```python
from build123d import *

# Parameters (mm, degrees)
F1_DEPTH = 5
F2_W     = 10
F2_H     = 4
F3_DEPTH = 25
F4_R     = 5
F5_R     = 5


with BuildPart() as f1:
    # F0 (on Front) → F1 (new body)
    with BuildSketch(Plane.XZ):
        with BuildLine():
            Line((-60, -80), (-60, 0))
            Line((-60, 0), (0, 0))
            Line((0, 0), (60, 0))
            Line((60, 0), (60, -80))
            ThreePointArc((60, -80), (62.5, -82.5), (65, -80))
            Line((65, -80), (65, 8))
            Line((65, 8), (60, 8))
            Line((60, 8), (43, 8))
            Line((43, 8), (43, 32.420063))
            ThreePointArc((43, 32.420063), (40.5, 34.920063), (38, 32.420063))
            Line((38, 32.420063), (38, 15.420063))
            Line((38, 15.420063), (35.5, 15.420063))
            Line((35.5, 15.420063), (35.5, 8))
            Line((35.5, 8), (0, 8))
            Line((0, 8), (-35.5, 8))
            Line((-35.5, 8), (-35.5, 15.420063))
            Line((-35.5, 15.420063), (-38, 15.420063))
            Line((-38, 15.420063), (-38, 32.420063))
            ThreePointArc((-38, 32.420063), (-40.5, 34.920063), (-43, 32.420063))
            Line((-43, 32.420063), (-43, 8))
            Line((-43, 8), (-60, 8))
            Line((-60, 8), (-65, 8))
            Line((-65, 8), (-65, -80))
            ThreePointArc((-65, -80), (-62.5, -82.5), (-60, -80))
        make_face()
    extrude(amount=F1_DEPTH)

    # F2 (on Front) → F3 (cut)
    with BuildSketch(Plane.XZ):
        with Locations((0, 8)):
            Rectangle(F2_W, F2_H)
    extrude(amount=F3_DEPTH, mode=Mode.SUBTRACT)

    # F4
    f4_edges = [f1.edges().sort_by_distance(p)[0] for p in [
        (-65, -2.5, 8),
        (65, -2.5, 8),
    ]]
    fillet(f4_edges, radius=F4_R)

    # F5
    f5_edges = [f1.edges().sort_by_distance(p)[0] for p in [
        (-43, -2.5, 8),
        (43, -2.5, 8),
    ]]
    fillet(f5_edges, radius=F5_R)


solid = f1.part
```
Geometry: final body of the model. Coordinates: model frame, mm. A direction names the side the tool comes from. Give positions to 0.01 mm unless a question says otherwise; leave off trailing zeros. Write each loop counter-clockwise with the first axis right and the second up, starting at its lowest first coordinate (ties: lowest second). Pieces come first, ordered by that corner, then holes.
1. Reachability of faces 4 (the flat face through (-54, -2, 8)), 5 (the flat face through (54, -2, 8)), 6 (the flat face through (-60, -2, -41)), 7 (the flat face through (-65, -2, -38)), 8 (the flat face through (35.5, -2, 12)) from +Z, -Z, +X, -X, +Y, -Y: full face, straight path, thin tool, end or side. Return the list, or none.
2. Section query B-B, the plane y = -3.2. Return loops of the section in (x, z).
3. Section query A-A, the plane z = -34. Return loops of the section in (x, y), then the cut area to 3 significant figures.
4. Section query D-D, the plane x = 62.5. Return loops of the section in (y, z), then the cut area to 3 significant figures.
5. Line query: probe 1 along X at (y, z) = (-4.2, -60); probe 2 along X at (y, z) = (-3.8, 19); probe 3 along Z at (x, y) = (-19, -2.25). Output: solid intervals per line, ascending.
6. Section query C-C, the plane x = -52. Return loops of the section in (y, z), then the cut area to 3 significant figures.
7. Draft query along Y for faces 1 (the flat face through (0, 0, 3)), 2 (the flat face through (0, -2, 6)), 3 (the flat face through (0, -5, 3)). Return one class per face: released by +Y, released by -Y, zero draft, split by the parting line, or undercut.
8. Pin query (flat end, axial travel): P1, Ø2.5, axis at x = 1.5, y = -2.5, coming from the +Z side; P2, Ø2, axis at y = -2, z = 13, coming from the -X side; P3, Ø2.5, axis at y = -3.5, z = 18, coming from the -X side. Return the tip coordinate at first contact, or that it passes through.
Computed:
1. face 4: +Z, -X, +Y, -Y
1. face 5: +Z, +X, +Y, -Y
1. face 6: -Z, +Y, -Y
1. face 7: +Z, -Z, -X, +Y, -Y
1. face 8: +Z, +Y, -Y
2. outline: (-65, -80) arc R2.5 ccw to (-60, -80) - (-60, 0) - (60, 0) - (60, -80) arc R2.5 ccw to (65, -80) - (65, 3) arc R5 ccw to (60, 8) - (48, 8) arc R5 cw to (43, 13) - (43, 32.42) arc R2.5 ccw to (38, 32.42) - (38, 15.42) - (35.5, 15.42) - (35.5, 8) - (5, 8) - (5, 6) - (-5, 6) - (-5, 8) - (-35.5, 8) - (-35.5, 15.42) - (-38, 15.42) - (-38, 32.42) arc R2.5 ccw to (-43, 32.42) - (-43, 13) arc R5 cw to (-48, 8) - (-60, 8) arc R5 ccw to (-65, 3) - close
3. outline: (-65, -5) - (-60, -5) - (-60, 0) - (-65, 0) - close; (60, -5) - (65, -5) - (65, 0) - (60, 0) - close
3. area: 50.0 mm2
4. outline: (-5, -82.5) - (0, -82.5) - (0, 7.33) - (-5, 7.33) - close
4. area: 449 mm2
5. probe 1: x = -65 to -60, 60 to 65
5. probe 2: x = -43 to -38, 38 to 43
5. probe 3: z = 0 to 8
6. outline: (-5, 0) - (0, 0) - (0, 8) - (-5, 8) - close
6. area: 40.0 mm2
7. face 1: released by +Y
7. face 2: zero draft
7. face 3: released by -Y
8. P1: stops at z = 6
8. P2: stops at x = -43.1
8. P3: stops at x = -43
